```python
from build123d import *

# Parameters (mm, degrees)
SKETCH002_R             = 2.6
PAD001_DEPTH            = 2
PAD002_DEPTH            = 2
POCKET003_DEPTH         = 2.201
PAD003_DEPTH            = 2.2
POCKET004_DEPTH         = 4.001
SKETCH006_R             = 17.1
SKETCH006_R_2           = 14.9
POCKET002_DEPTH         = 1
CHAMFER002_SIZE         = 0.4
CHAMFER_SIZE            = 1.99
SKETCH004_R             = 2.2
POCKET_DEPTH            = 4.001
SKETCH005_R             = 6.2
POCKET001_DEPTH         = 2.001
SKETCH010_R             = 4
POCKET005_DEPTH         = 1
CHAMFER001_SIZE         = 1.7
BODY002_PLACEMENT_ANGLE = 120


with BuildPart() as part:
    # Sketch002 → Pad001 (new body)
    with BuildSketch(Plane.XY):
        Polygon((-116.824546, 67.621888), (-37.5, 205.016032), (37.5, 205.016032), (116.824546, 67.621888), (0, 0.173205), align=None)
        with Locations((-51.370835, 167.991041)):
            Circle(SKETCH002_R, mode=Mode.SUBTRACT)
        with Locations((51.370835, 167.991041)):
            Circle(SKETCH002_R, mode=Mode.SUBTRACT)
    extrude(amount=PAD001_DEPTH)

    # Sketch003 → Pad002 (join)
    with BuildSketch(Plane.XY.offset(2)):
        Polygon((-118.899546, 64.027883), (-114.899546, 70.956086), (-0.173205, 4.718802), (-0.173205, 0.1), (-4.173205, -2.209401), align=None)
    extrude(amount=PAD002_DEPTH)

    # Sketch007 → Pocket003 (cut, through all)
    with BuildSketch(Plane.XY.offset(2.2)):
        Polygon((-116.824546, 67.621888), (0, 0.173205), (-4.173205, -2.209401), (-118.899546, 64.027883), align=None)
    extrude(amount=-POCKET003_DEPTH, mode=Mode.SUBTRACT)

    # Sketch008 → Pad003 (join)
    with BuildSketch(Plane.XY):
        Polygon((-104.909165, 58.259933), (-87.588657, 48.259933), (-88.588657, 46.527883), (-105.909165, 56.527883), align=None)
    extrude(amount=PAD003_DEPTH)

    # Sketch009 → Pocket004 (cut, through all)
    with BuildSketch(Plane.XY):
        Polygon((83.830836, 53.168669), (84.960836, 51.211452), (103.666985, 62.011452), (102.536985, 63.968669), align=None)
    extrude(amount=POCKET004_DEPTH, mode=Mode.SUBTRACT)

    # Sketch006 → Pocket002 (cut)
    with BuildSketch(Plane.XY):
        Circle(SKETCH006_R)
        Circle(SKETCH006_R_2, mode=Mode.SUBTRACT)
    extrude(amount=POCKET002_DEPTH, mode=Mode.SUBTRACT)

    # Chamfer002
    chamfer002_edges = [part.edges().sort_by_distance(p)[0] for p in [
        (-96.248911, 53.259933, 0),
        (-88.088657, 47.393908, 0),
        (-97.248911, 51.527883, 0),
        (-105.409165, 57.393908, 0),
        (94.313911, 56.611452, 0),
        (103.101985, 62.99006, 0),
        (93.183911, 58.568669, 0),
        (84.395836, 52.19006, 0),
        (0, 14.9, 0),
        (0, 17.1, 0),
    ]]
    chamfer(chamfer002_edges, length=CHAMFER002_SIZE)

    # Chamfer
    chamfer_edges = [part.edges().sort_by_distance(p)[0] for p in [
        (-57.536375, 37.837444, 4),
    ]]
    chamfer(chamfer_edges, length=CHAMFER_SIZE)

    # Sketch004 → Pocket (cut, through all)
    with BuildSketch(Plane.XY):
        Circle(SKETCH004_R)
    extrude(amount=POCKET_DEPTH, mode=Mode.SUBTRACT)

    # Sketch005 → Pocket001 (cut, through all)
    with BuildSketch(Plane.XY.offset(2)):
        Circle(SKETCH005_R)
    extrude(amount=POCKET001_DEPTH, mode=Mode.SUBTRACT)

    # Sketch010 → Pocket005 (cut)
    with BuildSketch(Plane.XY.offset(2)):
        with Locations((-51.370835, 167.991041)):
            Circle(SKETCH010_R)
        with Locations((51.370835, 167.991041)):
            Circle(SKETCH010_R)
    extrude(amount=-POCKET005_DEPTH, mode=Mode.SUBTRACT)

    # Chamfer001
    chamfer001_edges = [part.edges().sort_by_distance(p)[0] for p in [
        (-5.849077, 2.056283, 4),
        (-62.500992, 31.466162, 4),
        (-117.397046, 66.630289, 4),
    ]]
    chamfer(chamfer001_edges, length=CHAMFER001_SIZE)


with BuildPart() as part_1:
    # Body002 placement: moved
    add(part.part.rotate(Axis((0, 0, 0), (0, 0, 1)), BODY002_PLACEMENT_ANGLE))


solid = part_1.part
```
Model file for the job. Use its own axes, mm. A direction names the side the tool comes from. Coordinates: 2 decimals unless noted, no trailing zeros. Loops run counter-clockwise (first coordinate to the right, second up) from the corner with the lowest first, then second, coordinate; pieces in that order, holes last. Notation, with made-up numbers: (-2.5, 85.5) - (56.5, 85.5) arc R35 cw to (56.5, 118.5) - close; hole circle Ø1 at (47, 40). An arc over 180 degrees is marked (long way). Answer as a JSON object with one key per item and string values. Group by question number.
(1) Flat gauge pins, fed straight in: pin 1 (1.4 mm diameter, centred on y = -105.5, z = 1, fed in from -X); pin 2 (1 mm diameter, centred on x = -140, z = 2, fed in from +Y); pin 3 (7 mm diameter, centred on x = -171.17, y = -39.51, fed in from +Z). Where does each tip first touch, or does it go through?
(2) Cut at B-B (x = -146). Give the cut face in (y, z).
(3) Probe line 1 along Z through (x, y) = (-124, -107); line 2 along X through (y, z) = (-74, 2.85); line 3 along X through (y, z) = (-59, 3.8). List the from-to ranges inside material, lowest first.
(4) Tool access for faces 1 (the face through (-97.44, 51.49, 1.19)), 2 (the face through (-167.355, -38.306, 1.507)), 3 (the face through (-14, -7, 1)), 4 (the face through (0, -70, 4)): list every direction of +Z, -Z, +X, -X, +Y, -Y with a clear straight run to the whole face (end or side of a thin tool).
(5) Two-plate mould, pull along X, no slides. Class faces 5 (the face through (-60.28, 34.63, 0.99)), 6 (the face through (-96.053, 53.297, 1.189)), 7 (the face through (-92, -50, 2)): released by +X, released by -X, zero draft, split by the parting line, or undercut.
(6) Cut at D-D (x = -35). Give the cut face in (y, z), then the cut area to 3 significant figures.
Geometry says:
{
 "1": {"pin 1": "stops at x = -176.23", "pin 2": "stops at y = 28.35", "pin 3": "stops at z = 1"},
 "2": {"outline": "(-134.98, 0) - (17.09, 0) - (17.09, 2) - (-134.98, 2) - close"},
 "3": {"line 1": "z = 0 to 2", "line 2": "x = -3.16 to 3.45", "line 3": "x = -2.21 to 2.5"},
 "4": {"face 1": "+Z, -Z", "face 2": "+Z", "face 3": "-Z", "face 4": "+Z, +X, -X, +Y, -Y"},
 "5": {"face 5": "released by +X", "face 6": "undercut", "face 7": "zero draft"},
 "6": {"outline": "(-134.98, 0) - (20.03, 0) - (20.03, 2) - (-134.98, 2) - close", "area": "310 mm^2"}
}
